```python
from build123d import *

# Parameters (mm, degrees)
BODY_DEPTH = 9.4234


with BuildPart() as part:
    # BodySke → Body (new body)
    with BuildSketch(Plane(origin=(0, 0, 0), x_dir=(0, 0, -1), z_dir=(1, 0, 0))):
        with BuildLine():
            Line((-5.8674, -9.525), (5.8674, -9.525))
            Line((5.8674, -9.525), (5.8674, -8.9154))
            Line((5.8674, -8.9154), (4.8514, -8.9154))
            Line((4.8514, -8.9154), (4.8514, -8.6106))
            Line((4.8514, -8.6106), (5.1054, -8.6106))
            Line((5.1054, -8.6106), (5.1054, -8.001))
            Line((5.1054, -8.001), (4.504485143, -6.35))
            Line((4.504485143, -6.35), (3.520438226, -6.35))
            ThreePointArc((3.520438226, -6.35), (2.069125842, -5.296760115), (2.620488612, -3.59041285))
            ThreePointArc((2.620488612, -3.59041285), (4.442829508, 0.138891913), (2.391103448, 3.747085441))
            Line((2.391103448, 3.747085441), (0.9906, 1.552363968))
            ThreePointArc((0.9906, 1.552363968), (0, -1.8415), (-0.9906, 1.552363968))
            Line((-0.9906, 1.552363968), (-2.391103448, 3.747085441))
            ThreePointArc((-2.391103448, 3.747085441), (-4.442829508, 0.138891913), (-2.620488612, -3.59041285))
            ThreePointArc((-2.620488612, -3.59041285), (-2.069125842, -5.296760115), (-3.520438226, -6.35))
            Line((-3.520438226, -6.35), (-4.504485143, -6.35))
            Line((-4.504485143, -6.35), (-5.1054, -8.001))
            Line((-5.1054, -8.001), (-5.1054, -8.6106))
            Line((-5.1054, -8.6106), (-4.8514, -8.6106))
            Line((-4.8514, -8.6106), (-4.8514, -8.9154))
            Line((-4.8514, -8.9154), (-5.8674, -8.9154))
            Line((-5.8674, -8.9154), (-5.8674, -9.525))
        make_face()
    extrude(amount=BODY_DEPTH)


solid = part.part
```
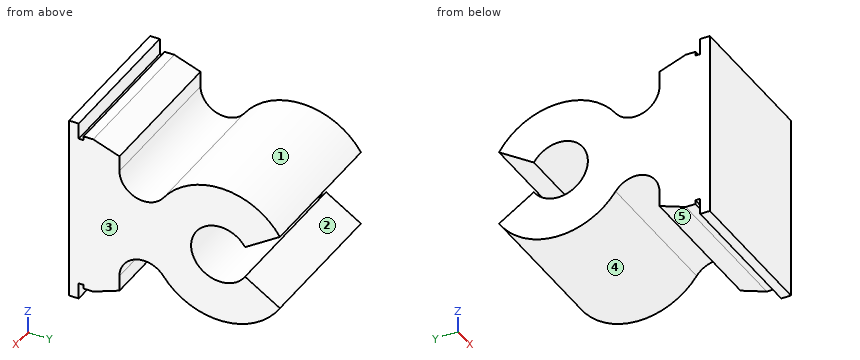
CAD build for the part. Positions are in the model's coordinates, mm. Face numbers are marked on the shaded views. A direction names the side the tool comes from. Coordinates: 2 decimals unless noted, no trailing zeros. Order: outer loops, then holes, each group sorted by start corner. A loop starts at its lowest first (then second) coordinate and runs counter-clockwise, first axis right, second up. Notation, with made-up numbers: (50.25, 24) -> (103.25, 24) arc R20 cw to (103.25, 43) -> close; hole circle Ø5 at (36, -25.75). An arc over 180 degrees is marked (long way). Use one line per item in the form item = value. Start each with the question number.
1) Pull direction Y, two halves, no side cores. Call the marked faces 3, 4 and 5: +Y half, -Y half, draft (parallel to the pull), parting line (faces both ways), or undercut.
2) Drill centre lines: L1, parallel to Z at x = 4.5, y = 0 (1 decimal); L2, parallel to Z at x = 8.75, y = 2; L3, parallel to Y at x = 6, z = 2.5 (3 decimals). Where is each one in solid material? Low to high. Write a range as [from, to].
3) Band-saw the part on A-A on y = 0. Give the cut face in (x, z) (1 decimal), then the cut area to 3 significant figures.
4) Drop flat-ended pins along their axis: pin 1 (1.1 mm diameter, centred on x = 4, z = -4, fed in from +Y); pin 2 (0.8 mm diameter, centred on x = 5.5, z = 4, fed in from +Y); pin 3 (0.5 mm diameter, centred on x = 5.5, y = -8, fed in from -Z). Give the stop position or say it passes through.
5) Band-saw the part on B-B on z = -4. Give the cut face in (x, y) (3 decimals).
6) Band-saw the part on D-D on z = 0. Give the cut face in (x, y) (1 decimal).
7) Tool access for the marked faces 1 and 2: list every direction of +Z, -Z, +X, -X, +Y, -Y with a clear straight run to the whole face (end or side of a thin tool).
Entries:
q1.face_3 = draft
q1.face_4 = undercut
q1.face_5 = +Y half
q2.L1 = [-4.4, -1.8], [1.8, 4.4]
q2.L2 = [-3.97, -1.28], [1.28, 3.97]
q2.L3 = [-9.525, -5.959], [-3.688, 3.675]
q3.outline = (0, -4.4) -> (9.4, -4.4) -> (9.4, -1.8) -> (0, -1.8) -> close; (0, 1.8) -> (9.4, 1.8) -> (9.4, 4.4) -> (0, 4.4) -> close
q3.area = 49.1 mm2
q4.pin_1 = 2.8
q4.pin_2 = 2.61
q4.pin_3 = -5.11
q5.outline = (0, -9.525) -> (9.423, -9.525) -> (9.423, -6.35) -> (0, -6.35) -> close; (0, -1.939) -> (9.423, -1.939) -> (9.423, 1.939) -> (0, 1.939) -> close
q6.outline = (0, -9.5) -> (9.4, -9.5) -> (9.4, -1.8) -> (0, -1.8) -> close
q7.face_1 = +Z, +X, -X
q7.face_2 = +X, -X, +Y
